Answer from the drawing. Dimensions are ordinates in mm from the lowest x, y and z of the part. A direction names the side the tool comes from. Give positions to 0.01 mm unless a question says otherwise; leave off trailing zeros. Write each loop counter-clockwise with the first axis right and the second up, starting at its lowest first coordinate (ties: lowest second). Pieces come first, ordered by that corner, then holes. Notation, with made-up numbers: M 9.5,0 L 22.5,0 A26 ccw 22.5,25 Z; hole C 19.25,88.25 d5. An arc over 180 degrees is marked long. Answer as a JSON object with one key per item and string values.
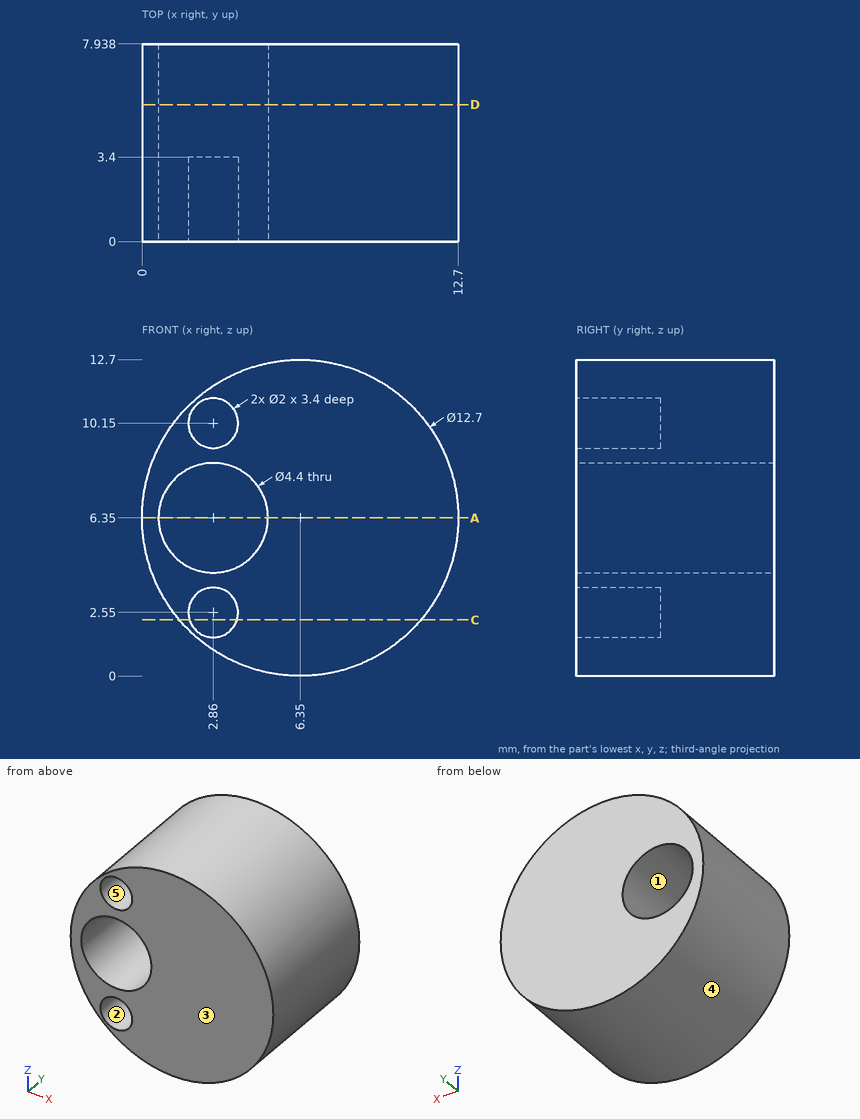
1. A cutting plane is placed at D-D, the plane y = 5.5. Give the vertices of the cut face in (x, z).
Verdict:
{"outline": "C 6.35,6.35 d12.7; hole C 2.86,6.35 d4.4"}
2. For the marked faces 1 and 2, determine the directions among +Z, -Z, +X, -X, +Y, -Y from which every point of the face is accessible in a straight line to the end or side of a thin tool.
Verdict:
{"face 1": "+Y, -Y", "face 2": "-Y"}
3. Flat-ended cylindrical pins translate along their axes: pin 1 (1.5 mm diameter, centred on x = 7, y = 6, fed in from -Z); pin 2 (1.8 mm diameter, centred on x = 2.86, z = 10.15, fed in from -Y); pin 3 (4 mm diameter, centred on x = 3.5, y = 2, fed in from +Z); pin 4 (4 mm diameter, centred on y = 3.5, z = 3, fed in from +X) (1 decimal). Find the tip coordinate at first contact, or state that the pin passes through.
Verdict:
{"pin 1": "stops at z = 0", "pin 2": "stops at y = 3.4", "pin 3": "stops at z = 12.64", "pin 4": "stops at x = 12.6"}
4. A cutting plane is placed at A-A, the plane z = 6.35. Give the vertices of the cut face in (x, y).
Verdict:
{"outline": "M 0,0 L 0.66,0 L 0.66,7.94 L 0,7.94 Z; M 5.06,0 L 12.7,0 L 12.7,7.94 L 5.06,7.94 Z"}
5. Consider line 1 along X through (y, z) = (3.5, 6.35); line 2 along Z through (x, y) = (2.25, 1.25) (1 decimal); line 3 along X through (y, z) = (1.35, 10.15) (1 decimal). Determine where each line is inside the solid, lowest interval first.
Verdict:
{"line 1": "x = 0 to 0.66, 5.06 to 12.7", "line 2": "z = 1.5 to 1.8, 3.3 to 4.2, 8.5 to 9.4, 10.9 to 11.2", "line 3": "x = 1.3 to 1.9, 3.9 to 11.4"}
6. The mould has two halves that part along X. Classify the marked faces 3, 4 and 5: released by +X, released by -X, zero draft, split by the parting line, or undercut.
Verdict:
{"face 3": "zero draft", "face 4": "split by the parting line", "face 5": "undercut"}
7. A cutting plane is placed at C-C, the plane z = 2.25. Give the vertices of the cut face in (x, y).
Verdict:
{"outline": "M 1.5,0 L 1.91,0 L 1.91,3.4 L 3.81,3.4 L 3.81,0 L 11.2,0 L 11.2,7.94 L 1.5,7.94 Z"}
